Can you work these out from the model? Positions are in its coordinate system, mm. Face numbers are marked on the shaded views. A direction names the side the tool comes from. Give positions to 0.01 mm unless a question says otherwise; leave off trailing zeros. Order: outer loops, then holes, each group sorted by start corner. A loop starts at its lowest first (then second) coordinate and runs counter-clockwise, first axis right, second up.
Item 1: I want a section at C-C, the plane x = -17.5. Write out the boundary of the cut face in (y, z) (3 decimals).
Item 2: Which directions (+Z, -Z, +X, -X, +Y, -Y) give clear straight access to the entire face, cutting with the end or side of a thin tool? Please do the marked faces 1, 2 and 3.
Item 3: I want a section at A-A, the plane x = -76.2. Write out the boundary of the cut face in (y, z) (3 decimals), then the cut area to 3 significant figures.
Item 4: I want a section at D-D, the plane y = 68. Write out the boundary of the cut face in (x, z) (3 decimals), then the cut area to 3 significant figures.
Item 5: If I drill on line 1 along Z through (x, y) = (-76, 73) (3 decimals); line 2 along X through (y, z) = (-30.5, 0); line 3 along Y through (x, z) = (-19, 8) (3 decimals), over which ranges is the centre line in solid material (lowest first)?
Item 6: I'm going to push flat-ended pins straight in: pin 1 Ø5.5 at (x, y) = (-2, -40.5) entering from +Z; pin 2 Ø21 at (x, z) = (-77, 13) entering from -Y; pin 3 Ø8 at (x, z) = (0, 0) entering from -Y. Where does each tip first touch, or does it pass through?
Item 7: I want a section at B-B, the plane y = -10. Write out the boundary of the cut face in (x, z) (3 decimals), then the cut area to 3 significant figures.
Item 8: If we mould it in two halves opening along Z, with no side actions, what happens to the marked faces 4, 5, 6 and 7? For each: +Z half, -Z half, draft (parallel to the pull), parting line (faces both ways), or undercut.
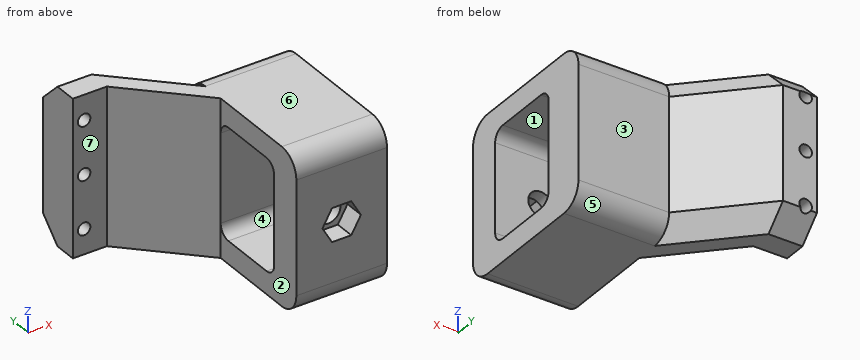
```python
from build123d import *

# Parameters (mm, degrees)
SKETCH002_W          = 87.63
SKETCH002_H          = 87.63
PAD001_DEPTH         = 25.4
FILLET002_R          = 12.065
SKETCH003_W          = 44.45
SKETCH003_H          = 62.23
POCKET001_DEPTH      = 25.401
POCKET001_DEPTH_BACK = 25.401
FILLET003_R          = 6.35
SKETCH004_R          = 6.85
POCKET002_DEPTH      = 18.416
POCKET003_DEPTH      = 11.176
PAD002_DEPTH         = 19.05
SKETCH008_R          = 3.5
POCKET004_DEPTH      = 24.766


with BuildPart() as part:
    # Sketch002 → Pad001 (new body, symmetric)
    with BuildSketch(Plane.YZ):
        Rectangle(SKETCH002_W, SKETCH002_H)
    extrude(amount=PAD001_DEPTH, both=True)

    # Fillet002
    fillet002_edges = [part.edges().sort_by_distance(p)[0] for p in [
        (0, -43.815, 43.815),
        (0, -43.815, -43.815),
        (0, 43.815, -43.815),
        (0, 43.815, 43.815),
    ]]
    fillet(fillet002_edges, radius=FILLET002_R)

    # Sketch003 → Pocket001 (cut, two sides)
    with BuildSketch(Plane.YZ) as pocket001_sk:
        with Locations((-3.175, 0)):
            Rectangle(SKETCH003_W, SKETCH003_H)
    extrude(amount=POCKET001_DEPTH, mode=Mode.SUBTRACT)
    extrude(pocket001_sk.sketch, amount=-POCKET001_DEPTH_BACK, mode=Mode.SUBTRACT)

    # Fillet003
    fillet003_edges = [part.edges().sort_by_distance(p)[0] for p in [
        (0, -25.4, -31.115),
        (0, 19.05, -31.115),
        (0, 19.05, 31.115),
        (0, -25.4, 31.115),
    ]]
    fillet(fillet003_edges, radius=FILLET003_R)

    # Sketch004 (on Face9 of Fillet003) → Pocket002 (cut, through all)
    with BuildSketch(Plane.ZX.offset(-25.4)):
        Circle(SKETCH004_R)
    extrude(amount=-POCKET002_DEPTH, mode=Mode.SUBTRACT)

    # Sketch005 (on Face13 of Pocket002) → Pocket003 (cut)
    with BuildSketch(Plane(origin=(0, -43.815, 0), x_dir=(0, 0, -1), z_dir=(0, -1, 0))):
        Polygon((9.348744, -5.3975), (9.348744, 5.3975), (0, 10.795), (-9.348744, 5.3975), (-9.348744, -5.3975), (0, -10.795), align=None)
    extrude(amount=-POCKET003_DEPTH, mode=Mode.SUBTRACT)

    # AdditivePipe: sweep along a path in Sketch007
    with BuildLine(Plane(origin=(0, 0, 43.815), x_dir=(0, -1, 0), z_dir=(0, 0, 1))) as additivepipe_path:
        Line((-31.75, -25.4), (-69.85, -63.5))
    # Sketch006 (on Face1 of Pocket003) → AdditivePipe (sweep)
    with BuildSketch(Plane(origin=(-25.4, 0, 0), x_dir=(0, 1, 0), z_dir=(-1, 0, 0))):
        Polygon((19.05, 43.815), (31.75, 43.815), (43.815, 31.75), (43.815, -31.75), (31.75, -43.815), (19.05, -43.815), (19.05, 24.765), align=None)
    sweep(path=additivepipe_path.line)

    # AdditivePipe Face20 → Pad002 (new)
    with BuildSketch(Plane(origin=(-63.5, 68.931373, 0), x_dir=(0, 1, 0), z_dir=(-1, 0, 0))):
        Polygon((-11.781373, -43.815), (0.918627, -43.815), (12.983627, -31.75), (12.983627, 31.75), (0.918627, 43.815), (-11.781373, 43.815), (-11.781373, 24.765), align=None)
    extrude(amount=PAD002_DEPTH)

    # Sketch008 (on Face20 of Pad002) → Pocket004 (cut, through all)
    with BuildSketch(Plane(origin=(0, 57.15, 0), x_dir=(0, 0, -1), z_dir=(0, -1, 0))):
        with Locations((-29.845, -76.2)):
            Circle(SKETCH008_R)
        with Locations((0, -76.2)):
            Circle(SKETCH008_R)
        with Locations((29.845, -76.2)):
            Circle(SKETCH008_R)
    extrude(amount=-POCKET004_DEPTH, mode=Mode.SUBTRACT)


solid = part.part
```
Results list:
1. outline: (-43.815, -31.75) arc R12.065 ccw to (-31.75, -43.815) - (31.75, -43.815) arc R12.065 ccw to (43.815, -31.75) - (43.815, 31.75) arc R12.065 ccw to (31.75, 43.815) - (-31.75, 43.815) arc R12.065 ccw to (-43.815, 31.75) - close; hole (-25.4, -24.765) arc R6.35 ccw to (-19.05, -31.115) - (12.7, -31.115) arc R6.35 ccw to (19.05, -24.765) - (19.05, 24.765) arc R6.35 ccw to (12.7, 31.115) - (-19.05, 31.115) arc R6.35 ccw to (-25.4, 24.765) - close
2. face 1: +X, -X
2. face 2: +Z, -Z, -X, -Y
2. face 3: +Z, -Z, +X, +Y
3. outline: (57.15, -43.815) - (69.85, -43.815) - (80.32, -33.345) - (57.15, -33.345) - close; (57.15, -26.345) - (81.915, -26.345) - (81.915, -3.5) - (57.15, -3.5) - close; (57.15, 3.5) - (81.915, 3.5) - (81.915, 26.345) - (57.15, 26.345) - close; (57.15, 33.345) - (80.32, 33.345) - (69.85, 43.815) - (57.15, 43.815) - close
3. area: 1,510 mm2
4. outline: (-82.55, -43.815) - (-61.65, -43.815) - (-49.585, -31.75) - (-49.585, 31.75) - (-61.65, 43.815) - (-82.55, 43.815) - close; hole circle Ø7 at (-76.2, -29.845); hole circle Ø7 at (-76.2, 0); hole circle Ø7 at (-76.2, 29.845)
4. area: 2,630 mm2
5. line 1: z = -40.665 to -33.339, -26.351 to -3.494, 3.494 to 26.351, 33.339 to 40.665
5. line 2: x = -25.4 to -6.85, 6.85 to 25.4
5. line 3: y = -43.815 to -25.4, 19.05 to 43.815
6. pin 1: stops at z = 42.22
6. pin 2: stops at y = 57.15
6. pin 3: stops at y = 19.05
7. outline: (-25.4, -43.815) - (25.4, -43.815) - (25.4, -31.115) - (-25.4, -31.115) - close; (-25.4, 31.115) - (25.4, 31.115) - (25.4, 43.815) - (-25.4, 43.815) - close
7. area: 1,290 mm2
8. face 4: undercut
8. face 5: -Z half
8. face 6: +Z half
8. face 7: draft
